```python
from build123d import *

# Parameters (mm, degrees)
BOSS_EXTRUDE1_DEPTH = 2
BOSS_EXTRUDE2_DEPTH = 4
SKETCH3_W           = 28.1
SKETCH3_H           = 7.3
CUT_EXTRUDE1_DEPTH  = 4
FILLET1_R           = 2


with BuildPart() as part:
    # Sketch1 → Boss-Extrude1 (new body)
    with BuildSketch(Plane(origin=(0, 0, 0), x_dir=(1, 0, 0), z_dir=(0, 1, 0))):
        with BuildLine():
            Line((-19.5, 10.5), (19.5, 10.5))
            ThreePointArc((19.5, 10.5), (23.035533906, 9.035533906), (24.5, 5.5))
            Line((24.5, 5.5), (24.5, -5.5))
            ThreePointArc((24.5, -5.5), (23.035533906, -9.035533906), (19.5, -10.5))
            Line((19.5, -10.5), (-19.5, -10.5))
            ThreePointArc((-19.5, -10.5), (-23.035533906, -9.035533906), (-24.5, -5.5))
            Line((-24.5, -5.5), (-24.5, 5.5))
            ThreePointArc((-24.5, 5.5), (-23.035533906, 9.035533906), (-19.5, 10.5))
        make_face()
    extrude(amount=BOSS_EXTRUDE1_DEPTH)

    # Sketch2 → Boss-Extrude2 (add)
    with BuildSketch(Plane.XZ):
        with BuildLine():
            Line((-22.4, 5.5), (-22.4, -5.5))
            ThreePointArc((-22.4, -5.5), (-21.550609665, -7.550609665), (-19.5, -8.4))
            Line((-19.5, -8.4), (19.5, -8.4))
            ThreePointArc((19.5, -8.4), (21.550609665, -7.550609665), (22.4, -5.5))
            Line((22.4, -5.5), (22.4, 5.5))
            ThreePointArc((22.4, 5.5), (21.550609665, 7.550609665), (19.5, 8.4))
            Line((19.5, 8.4), (-19.5, 8.4))
            ThreePointArc((-19.5, 8.4), (-21.550609665, 7.550609665), (-22.4, 5.5))
        make_face()
        with BuildLine():
            Line((-20.9, 5.5), (-20.9, -5.5))
            ThreePointArc((-20.9, -5.5), (-20.489949494, -6.489949494), (-19.5, -6.9))
            Line((-19.5, -6.9), (19.5, -6.9))
            ThreePointArc((19.5, -6.9), (20.489949494, -6.489949494), (20.9, -5.5))
            Line((20.9, -5.5), (20.9, 5.5))
            ThreePointArc((20.9, 5.5), (20.489949494, 6.489949494), (19.5, 6.9))
            Line((19.5, 6.9), (-19.5, 6.9))
            ThreePointArc((-19.5, 6.9), (-20.489949494, 6.489949494), (-20.9, 5.5))
        make_face(mode=Mode.SUBTRACT)
    extrude(amount=BOSS_EXTRUDE2_DEPTH)

    # Sketch3 → Cut-Extrude1 (cut)
    with BuildSketch(Plane(origin=(0, 2, 0), x_dir=(1, 0, 0), z_dir=(0, 1, 0))):
        with Locations((0, 0.5)):
            Rectangle(SKETCH3_W, SKETCH3_H)
    extrude(amount=-CUT_EXTRUDE1_DEPTH, mode=Mode.SUBTRACT)

    # Fillet1
    fillet1_edges = [part.edges().sort_by_distance(p)[0] for p in [
        (-23.035533906, 2, -9.035533906),
        (0, 2, -10.5),
        (23.035533906, 2, -9.035533906),
        (24.5, 2, 0),
        (23.035533906, 2, 9.035533906),
        (0, 2, 10.5),
        (-23.035533906, 2, 9.035533906),
        (-24.5, 2, 0),
    ]]
    fillet(fillet1_edges, radius=FILLET1_R - 0.0001)  # a hair under: the kernel refuses the full size


solid = part.part
```
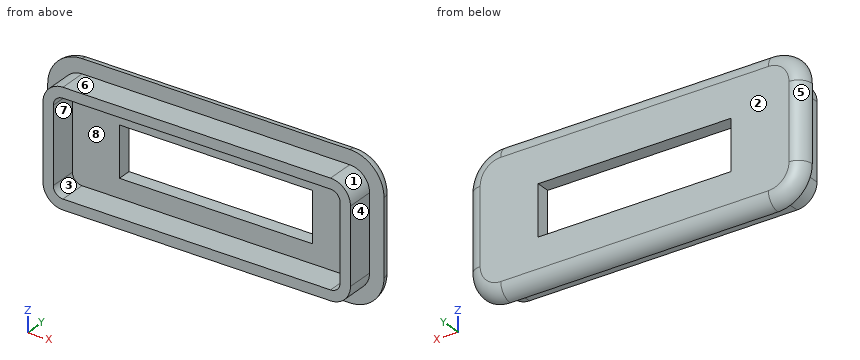
Design review of the part built by this model. Coordinates are the model's own, in mm. Face numbers are marked on the shaded views. A direction names the side the tool comes from. Coordinates: 2 decimals unless noted, no trailing zeros. Write each loop counter-clockwise with the first axis right and the second up, starting at its lowest first coordinate (ties: lowest second). Pieces come first, ordered by that corner, then holes.
1) Add section C-C (y = -3.25). Write out the cut boundary in (x, z).
2) Machinability: for the marked faces 1, 2, 3 and 4, which of the approach directions +Z, -Z, +X, -X, +Y, -Y give a long, thin tool a straight path to every point of the face, cutting with its end or side? Answer none if there is none.
3) To check wall thickness, follow L1, parallel to Z at x = 5.5, y = -1.6; L2, parallel to X at y = -3.1, z = 1.5; L3, parallel to Z at x = -13.5, y = 0.05. State the ranges of each line that lie inside material, in increasing order.
4) Insertion check: pin 1 (1.2 mm diameter, centred on y = -2, z = 2, fed in from +X); pin 2 (4 mm diameter, centred on x = -8, z = 0.5, fed in from -Y); pin 3 (3 mm diameter, centred on x = 5.5, y = -2, fed in from -Z); pin 4 (0.6 mm diameter, centred on y = 1, z = -1, fed in from +X). Each pin has a flat end and moves straight along its axis. Give the tip position at first contact, or say it passes through.
5) Mouldability with a two-part tool opening along Z and no side actions: class the marked faces 5, 6, 7 and 8 as +Z half, -Z half, draft (parallel to the pull), parting line (faces both ways), or undercut.
Check result:
1. outline: (-22.4, -5.5) arc R2.9 ccw to (-19.5, -8.4) - (19.5, -8.4) arc R2.9 ccw to (22.4, -5.5) - (22.4, 5.5) arc R2.9 ccw to (19.5, 8.4) - (-19.5, 8.4) arc R2.9 ccw to (-22.4, 5.5) - close; hole (-20.9, -5.5) arc R1.4 ccw to (-19.5, -6.9) - (19.5, -6.9) arc R1.4 ccw to (20.9, -5.5) - (20.9, 5.5) arc R1.4 ccw to (19.5, 6.9) - (-19.5, 6.9) arc R1.4 ccw to (-20.9, 5.5) - close
2. face 1: +Z, +X, -Y
2. face 2: +Z, -Z, +X, -X, +Y
2. face 3: -Y
2. face 4: +Z, -Z, +X, -Y
3. L1: z = -8.4 to -6.9, 6.9 to 8.4
3. L2: x = -22.4 to -20.9, 20.9 to 22.4
3. L3: z = -10.5 to -4.15, 3.15 to 10.5
4. pin 1: stops at x = 22.4
4. pin 2: passes through
4. pin 3: stops at z = -8.4
4. pin 4: stops at x = 24.37
5. face 5: draft
5. face 6: +Z half
5. face 7: undercut
5. face 8: undercut
